Build history of the part. All positions in model axes, mm. Coordinates: 2 decimals unless noted, no trailing zeros. Write each loop counter-clockwise with the first axis right and the second up, starting at its lowest first coordinate (ties: lowest second). Pieces come first, ordered by that corner, then holes. Notation, with made-up numbers: (72.25, 12) -> (110.25, 12) arc R28 cw to (110.25, 46) -> close; hole circle Ø1 at (69.5, 7.5). An arc over 180 degrees is marked (long way). Write each question's results on one line, items separated by ' | '. Start each with the question number.
Q1. Drop a flat-ended pin along its axis: pin 1 Ø3.5 at (x, z) = (25.98, 15) entering from +Y. Give the stop position or say it passes through.
Q2. Saw through at C-C on z = 15.5. Give the cut face in (x, y).
Q3. Saw through at D-D on y = 2.3. Count the separate pieces of the cut face and the enclosed holes in it, and give its area (3 significant figures).
Q4. Saw through at B-B on x = 34. Give the cut face in (y, z), and give its area (3 significant figures).
Q5. Drill centre lines: line 1 (X direction, y = 1.2, z = 15); line 2 (X direction, y = 2, z = 44.5); line 3 (X direction, y = 0.45, z = -10.5). Where is each one in solid material? Low to high.
Q6. Two-plate mould, pull along Z, no slides. Class faces 1 (the face through (-12.211, 1.521, -27.074)), 2 (the face through (-11, 3, 11)): released by +Z, released by -Z, zero draft, split by the parting line, or undercut.
Q7. Saw through at A-A on x = 0. Give the cut face in (y, z) (3 decimals), and give its area (3 significant figures).
from build123d import *

# Parameters (mm, degrees)
SKETCH_1_R          = 55
SKETCH_1_R_2        = 11.5
SKETCH_1_R_3        = 2.075
SKETCH_1_R_4        = 1.6
EXTRUDE_1_DEPTH     = 3
CUT_EXTRUDE_1_REACH = 79.84
FILLET_1_R          = 2


with BuildPart() as part:
    # 草图1 → 凸台-拉伸1 (new body)
    with BuildSketch(Plane(origin=(0, 0, 0), x_dir=(1, 0, 0), z_dir=(0, 1, 0))):
        with Locations(Location((0, 0, 0), (0, 0, 270))):
            Circle(SKETCH_1_R)
        with Locations(Location((0, 0, 0), (0, 0, 270))):
            Circle(SKETCH_1_R_2, mode=Mode.SUBTRACT)
        with Locations(Location((0, 30, 0), (0, 0, 270))):
            Circle(SKETCH_1_R_3, mode=Mode.SUBTRACT)
        with Locations(Location((25.980762114, -15, 0), (0, 0, 270))):
            Circle(SKETCH_1_R_3, mode=Mode.SUBTRACT)
        with Locations(Location((-25.980762114, -15, 0), (0, 0, 270))):
            Circle(SKETCH_1_R_3, mode=Mode.SUBTRACT)
        with Locations(Location((25, 43.301270189, 0), (0, 0, 270))):
            Circle(SKETCH_1_R_4, mode=Mode.SUBTRACT)
        with Locations(Location((50, 0, 0), (0, 0, 270))):
            Circle(SKETCH_1_R_4, mode=Mode.SUBTRACT)
        with Locations(Location((25, -43.301270189, 0), (0, 0, 270))):
            Circle(SKETCH_1_R_4, mode=Mode.SUBTRACT)
        with Locations(Location((-25, -43.301270189, 0), (0, 0, 270))):
            Circle(SKETCH_1_R_4, mode=Mode.SUBTRACT)
        with Locations(Location((-50, 0, 0), (0, 0, 270))):
            Circle(SKETCH_1_R_4, mode=Mode.SUBTRACT)
        with Locations(Location((-25, 43.301270189, 0), (0, 0, 270))):
            Circle(SKETCH_1_R_4, mode=Mode.SUBTRACT)
        with BuildLine():
            Line((-13.382612127, 14.86289651), (-28.772616073, 31.955227496))
            ThreePointArc((-28.772616073, 31.955227496), (-37.239092363, 21.5), (-42.060346832, 8.940202705))
            Line((-42.060346832, 8.940202705), (-19.562952015, 4.158233816))
            ThreePointArc((-19.562952015, 4.158233816), (-17.320508076, 10), (-13.382612127, 14.86289651))
        make_face(mode=Mode.SUBTRACT)
        with BuildLine():
            Line((19.562952015, 4.158233816), (42.060346832, 8.940202705))
            ThreePointArc((42.060346832, 8.940202705), (37.239092363, 21.5), (28.772616073, 31.955227496))
            Line((28.772616073, 31.955227496), (13.382612127, 14.86289651))
            ThreePointArc((13.382612127, 14.86289651), (17.320508076, 10), (19.562952015, 4.158233816))
        make_face(mode=Mode.SUBTRACT)
        with BuildLine():
            Line((-6.180339887, -19.021130326), (-13.287730758, -40.895430201))
            ThreePointArc((-13.287730758, -40.895430201), (0, -43), (13.287730758, -40.895430201))
            Line((13.287730758, -40.895430201), (6.180339887, -19.021130326))
            ThreePointArc((6.180339887, -19.021130326), (0, -20), (-6.180339887, -19.021130326))
        make_face(mode=Mode.SUBTRACT)
    extrude(amount=EXTRUDE_1_DEPTH)

    # 草图3 → 切除-拉伸1 (cut, up to next)
    with BuildSketch(Plane(origin=(0, 3, 0), x_dir=(1, 0, 0), z_dir=(0, 1, 0)), mode=Mode.PRIVATE) as cut_extrude_1_sk1:
        with BuildLine():
            Line((-20.66067252, 34.901813864), (-14.159583627, 27.68162318))
            ThreePointArc((-14.159583627, 27.68162318), (-12.181948481, 27.081178741), (-10.729018032, 28.551065609))
            Line((-10.729018032, 28.551065609), (-8.14424004, 39.270605536))
            ThreePointArc((-8.14424004, 39.270605536), (-8.682815659, 41.162100176), (-10.580638715, 41.677932823))
            ThreePointArc((-10.580638715, 41.677932823), (-15.454508197, 40.126776302), (-20.109718619, 38.007883617))
            ThreePointArc((-20.109718619, 38.007883617), (-21.143642812, 36.589381929), (-20.66067252, 34.901813864))
        make_face()
    cut_extrude_1_tool1 = extrude(cut_extrude_1_sk1.sketch, amount=-CUT_EXTRUDE_1_REACH, mode=Mode.PRIVATE) & part.part
    # 草图3 → 切除-拉伸1 (cut, up to next)
    with BuildSketch(Plane(origin=(0, 3, 0), x_dir=(1, 0, 0), z_dir=(0, 1, 0)), mode=Mode.PRIVATE) as cut_extrude_1_sk2:
        with BuildLine():
            Line((8.14424004, 39.270605536), (10.729018032, 28.551065609))
            ThreePointArc((10.729018032, 28.551065609), (12.181948481, 27.081178741), (14.159583627, 27.68162318))
            Line((14.159583627, 27.68162318), (20.66067252, 34.901813864))
            ThreePointArc((20.66067252, 34.901813864), (21.143642812, 36.589381929), (20.109718619, 38.007883617))
            ThreePointArc((20.109718619, 38.007883617), (15.454508197, 40.126776302), (10.580638715, 41.677932823))
            ThreePointArc((10.580638715, 41.677932823), (8.682815659, 41.162100176), (8.14424004, 39.270605536))
        make_face()
    cut_extrude_1_tool2 = extrude(cut_extrude_1_sk2.sketch, amount=-CUT_EXTRUDE_1_REACH, mode=Mode.PRIVATE) & part.part
    # 草图3 → 切除-拉伸1 (cut, up to next)
    with BuildSketch(Plane(origin=(0, 3, 0), x_dir=(1, 0, 0), z_dir=(0, 1, 0)), mode=Mode.PRIVATE) as cut_extrude_1_sk3:
        with BuildLine():
            Line((40.556193705, 0.441760329), (31.052780705, -1.578252462))
            ThreePointArc((31.052780705, -1.578252462), (29.543962994, -2.990712518), (30.090457138, -4.983930631))
            Line((30.090457138, -4.983930631), (38.081462036, -12.582183999))
            ThreePointArc((38.081462036, -12.582183999), (39.988832255, -13.061511152), (41.384467959, -11.675864496))
            ThreePointArc((41.384467959, -11.675864496), (42.478061748, -6.679391449), (42.970652066, -1.588414622))
            ThreePointArc((42.970652066, -1.588414622), (42.259155666, 0.016240839), (40.556193705, 0.441760329))
        make_face()
    cut_extrude_1_tool3 = extrude(cut_extrude_1_sk3.sketch, amount=-CUT_EXTRUDE_1_REACH, mode=Mode.PRIVATE) & part.part
    # 草图3 → 切除-拉伸1 (cut, up to next)
    with BuildSketch(Plane(origin=(0, 3, 0), x_dir=(1, 0, 0), z_dir=(0, 1, 0)), mode=Mode.PRIVATE) as cut_extrude_1_sk4:
        with BuildLine():
            Line((29.937221996, -26.688421537), (19.361439106, -23.567134977))
            ThreePointArc((19.361439106, -23.567134977), (17.362014513, -24.090466222), (16.893197078, -26.103370718))
            Line((16.893197078, -26.103370718), (19.895521185, -35.343574194))
            ThreePointArc((19.895521185, -35.343574194), (21.115512854, -36.605622768), (22.860933447, -36.419468995))
            ThreePointArc((22.860933447, -36.419468995), (27.023553551, -33.447384853), (30.803829244, -30.002068327))
            ThreePointArc((30.803829244, -30.002068327), (31.306016597, -28.100589025), (29.937221996, -26.688421537))
        make_face()
    cut_extrude_1_tool4 = extrude(cut_extrude_1_sk4.sketch, amount=-CUT_EXTRUDE_1_REACH, mode=Mode.PRIVATE) & part.part
    # 草图3 → 切除-拉伸1 (cut, up to next)
    with BuildSketch(Plane(origin=(0, 3, 0), x_dir=(1, 0, 0), z_dir=(0, 1, 0)), mode=Mode.PRIVATE) as cut_extrude_1_sk5:
        with BuildLine():
            Line((-19.895521185, -35.343574194), (-16.893197078, -26.103370718))
            ThreePointArc((-16.893197078, -26.103370718), (-17.362014513, -24.090466222), (-19.361439106, -23.567134977))
            Line((-19.361439106, -23.567134977), (-29.937221996, -26.688421537))
            ThreePointArc((-29.937221996, -26.688421537), (-31.306016597, -28.100589025), (-30.803829244, -30.002068327))
            ThreePointArc((-30.803829244, -30.002068327), (-27.023553551, -33.447384853), (-22.860933447, -36.419468995))
            ThreePointArc((-22.860933447, -36.419468995), (-21.115512854, -36.605622768), (-19.895521185, -35.343574194))
        make_face()
    cut_extrude_1_tool5 = extrude(cut_extrude_1_sk5.sketch, amount=-CUT_EXTRUDE_1_REACH, mode=Mode.PRIVATE) & part.part
    # 草图3 → 切除-拉伸1 (cut, up to next)
    with BuildSketch(Plane(origin=(0, 3, 0), x_dir=(1, 0, 0), z_dir=(0, 1, 0)), mode=Mode.PRIVATE) as cut_extrude_1_sk6:
        with BuildLine():
            Line((-38.081462036, -12.582183999), (-30.090457138, -4.983930631))
            ThreePointArc((-30.090457138, -4.983930631), (-29.543962994, -2.990712518), (-31.052780705, -1.578252462))
            Line((-31.052780705, -1.578252462), (-40.556193705, 0.441760329))
            ThreePointArc((-40.556193705, 0.441760329), (-42.259155666, 0.016240839), (-42.970652066, -1.588414622))
            ThreePointArc((-42.970652066, -1.588414622), (-42.478061748, -6.679391449), (-41.384467959, -11.675864496))
            ThreePointArc((-41.384467959, -11.675864496), (-39.988832255, -13.061511152), (-38.081462036, -12.582183999))
        make_face()
    cut_extrude_1_tool6 = extrude(cut_extrude_1_sk6.sketch, amount=-CUT_EXTRUDE_1_REACH, mode=Mode.PRIVATE) & part.part
    add(cut_extrude_1_tool1.solids().sort_by_distance((-13.924139, 3, -35.062692))[0], mode=Mode.SUBTRACT)
    add(cut_extrude_1_tool2.solids().sort_by_distance((13.924139, 3, -35.062692))[0], mode=Mode.SUBTRACT)
    add(cut_extrude_1_tool3.solids().sort_by_distance((37.327251, 3, 5.472688))[0], mode=Mode.SUBTRACT)
    add(cut_extrude_1_tool4.solids().sort_by_distance((23.403112, 3, 29.590004))[0], mode=Mode.SUBTRACT)
    add(cut_extrude_1_tool5.solids().sort_by_distance((-23.403112, 3, 29.590004))[0], mode=Mode.SUBTRACT)
    add(cut_extrude_1_tool6.solids().sort_by_distance((-37.327251, 3, 5.472688))[0], mode=Mode.SUBTRACT)

    # 圆角1
    fillet_1_edges = [part.edges().sort_by_distance(p)[0] for p in [
        (-28.772616073, 1.5, -31.955227496),
        (-42.060346832, 1.5, -8.940202705),
        (-19.562952015, 1.5, -4.158233816),
        (-13.382612127, 1.5, -14.86289651),
        (42.060346832, 1.5, -8.940202705),
        (28.772616073, 1.5, -31.955227496),
        (13.382612127, 1.5, -14.86289651),
        (19.562952015, 1.5, -4.158233816),
        (-13.287730758, 1.5, 40.895430201),
        (13.287730758, 1.5, 40.895430201),
        (6.180339887, 1.5, 19.021130326),
        (-6.180339887, 1.5, 19.021130326),
    ]]
    fillet(fillet_1_edges, radius=FILLET_1_R)


solid = part.part
Returned:
1) pin 1: passes through
2) outline: (-52.77, 0) -> (-27.99, 0) -> (-27.99, 3) -> (-52.77, 3) -> close; (-23.97, 0) -> (23.97, 0) -> (23.97, 3) -> (-23.97, 3) -> close; (27.99, 0) -> (52.77, 0) -> (52.77, 3) -> (27.99, 3) -> close
3) separate pieces: 1 | enclosed holes: 19 | area: 6,930 mm2
4) outline: (0, -43.23) -> (3, -43.23) -> (3, -26.32) -> (0, -26.32) -> close; (0, -7.23) -> (3, -7.23) -> (3, 0.95) -> (0, 0.95) -> close; (0, 8.7) -> (3, 8.7) -> (3, 43.23) -> (0, 43.23) -> close | area: 179 mm2
5) line 1: x = -52.92 to -28.06, -23.91 to 23.91, 28.06 to 52.92 | line 2: x = -32.32 to -26.06, -23.94 to 23.94, 26.06 to 32.32 | line 3: x = -53.99 to -41.64, -17.02 to -4.69, 4.69 to 17.02, 41.64 to 53.99
6) face 1: undercut | face 2: zero draft
7) outline: (0, -55) -> (3, -55) -> (3, -32.075) -> (0, -32.075) -> close; (0, -27.925) -> (3, -27.925) -> (3, -11.5) -> (0, -11.5) -> close; (0, 11.5) -> (3, 11.5) -> (3, 20) -> (0, 20) -> close; (0, 43) -> (3, 43) -> (3, 55) -> (0, 55) -> close | area: 180 mm2
